Can you work these out from the drawing? Everything is in mm from the part's minimum corner. A direction names the side the tool comes from. Coordinates: 2 decimals unless noted, no trailing zeros. Loops run counter-clockwise (first coordinate to the right, second up) from the corner with the lowest first, then second, coordinate; pieces in that order, holes last.
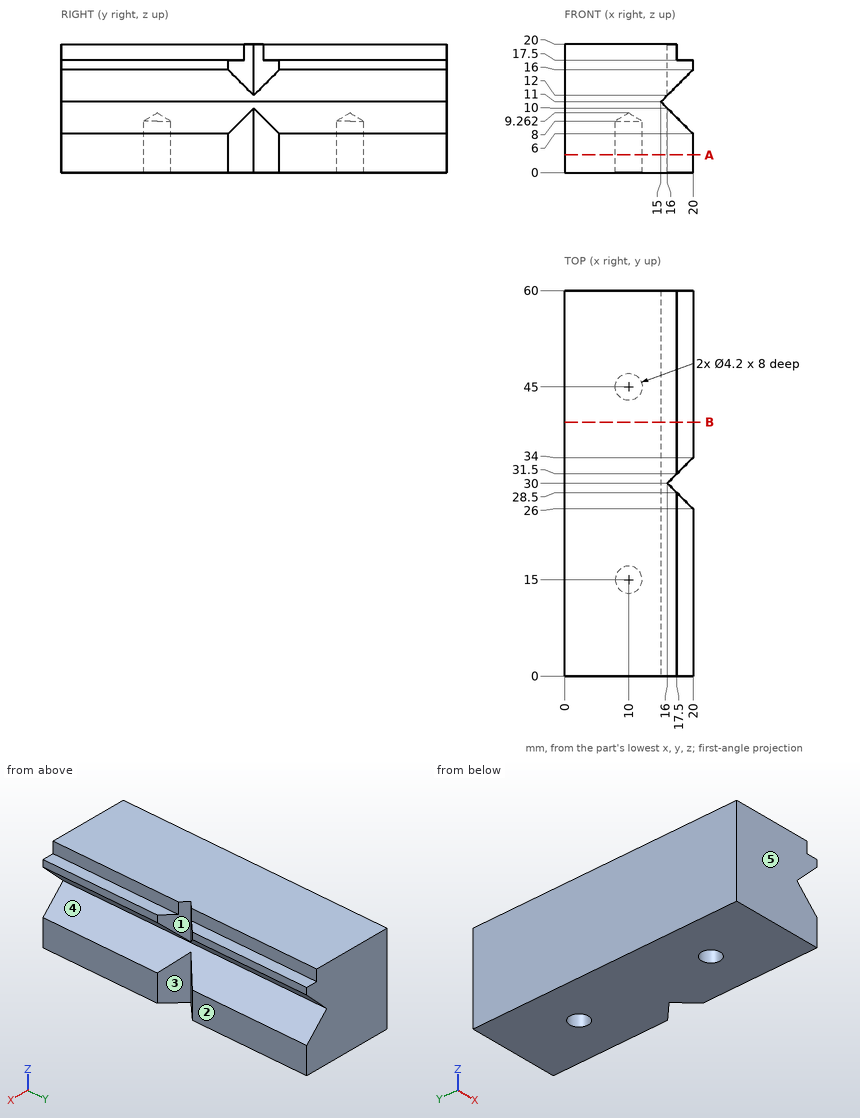
1. On a 3-axis mill with a long thin cutter (end or side, diameter ignored), from which of +Z, -Z, +X, -X, +Y, -Y can I reach the whole of each face in a straight line? I mean the marked faces 1 and 2. Say none if no direction works.
2. I want a section at B-B (y = 39.5). Please give me the cut outline in (x, z), then the cut area to 3 significant figures.
3. For pin 1 (1.2 mm diameter, centred on x = 18.5, y = 18, fed in from +Z); pin 2 (1 mm diameter, centred on x = 17, z = 9.5, fed in from -Y); pin 3 (2 mm diameter, centred on y = 46.5, z = 19, fed in from +X); pin 4 (2 mm diameter, centred on y = 23, z = 13, fed in from +X), each with a flat end and sliding along its axis, tell me the tip position at first contact or that it passes through.
4. We'd pull the mould along Y, two halves only. Please class the marked faces 3, 4 and 5: +Y half, -Y half, draft (parallel to the pull), parting line (faces both ways), or undercut.
5. I need wall thicknesses on line 1 along Y through (x, z) = (10, 4); line 2 along X through (y, z) = (45, 3.75); line 3 along X through (y, z) = (6.5, 19). Which ranges of each line are inside material? Lowest first, please.
6. I want a section at A-A (z = 2.75). Please give me the cut outline in (x, y).
Response values:
1. face 1: +Z, -Z, +X
1. face 2: +Z, -Z, +X, +Y, -Y
2. outline: (0, 0) - (20, 0) - (20, 6) - (15, 11) - (20, 16) - (20, 17.5) - (17.5, 17.5) - (17.5, 20) - (0, 20) - close
2. area: 369 mm2
3. pin 1: stops at z = 17.5
3. pin 2: stops at y = 0
3. pin 3: stops at x = 17.5
3. pin 4: stops at x = 18
4. face 3: undercut
4. face 4: draft
4. face 5: -Y half
5. line 1: y = 0 to 12.9, 17.1 to 42.9, 47.1 to 60
5. line 2: x = 0 to 7.9, 12.1 to 20
5. line 3: x = 0 to 17.5
6. outline: (0, 0) - (20, 0) - (20, 26) - (16, 30) - (20, 34) - (20, 60) - (0, 60) - close; hole circle Ø4.2 at (10, 15); hole circle Ø4.2 at (10, 45)
